```python
from build123d import *

# Parameters (mm, degrees)
ESBO_O2_W                  = 8.2
ESBO_O2_H                  = 30.460387467
RESSALTO_EXTRUS_O1_DEPTH   = 3
RESSALTO_EXTRUS_O1_2_DEPTH = 3
RESSALTO_EXTRUS_O2_REACH   = 32.935
ESBO_O3_W                  = 3
ESBO_O3_H                  = 6.088150409
ESBO_O4_W                  = 12.8
ESBO_O4_H                  = 2.7
RESSALTO_EXTRUS_O3_DEPTH   = 10
ESBO_O5_W                  = 8.2
ESBO_O5_H                  = 4.5
RESSALTO_EXTRUS_O4_DEPTH   = 16
CORTE_EXTRUS_O1_DEPTH      = 34.348189118
CORTE_EXTRUS_O1_DEPTH_BACK = 34.348189118
ESBO_O6_R                  = 1.6
ESBO_O7_R                  = 3
CORTE_EXTRUS_O2_DEPTH      = 2.5
ESBO_O8_R                  = 1.05
CORTE_EXTRUS_O3_DEPTH      = 32.131124741
FILETE1_R                  = 3
ESBO_O9_W                  = 1.2
ESBO_O9_H                  = 3.148787123
CORTE_EXTRUS_O4_DEPTH      = 2.7
FILETE2_R                  = 3
CORTE_EXTRUS_O5_DEPTH      = 1.8
ESBO_O13_W                 = 2.7
ESBO_O13_H                 = 3.148787123
CORTE_EXTRUS_O7_DEPTH      = 1.2


with BuildPart() as part:
    # Esbo_o2 → Ressalto-extrus_o1 (new body)
    with BuildSketch(Plane(origin=(0, 0, -1), x_dir=(-1, 0, 0), z_dir=(0, 0, -1))):
        with Locations((10.5, -7.130193734)):
            Rectangle(ESBO_O2_W, ESBO_O2_H)
    extrude(amount=RESSALTO_EXTRUS_O1_DEPTH)


with BuildPart() as body_2:
    # Esbo_o2 → Ressalto-extrus_o1 2 (new body)
    with BuildSketch(Plane(origin=(0, 0, -1), x_dir=(-1, 0, 0), z_dir=(0, 0, -1))):
        with Locations((-10.5, -7.130193734)):
            Rectangle(ESBO_O2_W, ESBO_O2_H)
    extrude(amount=RESSALTO_EXTRUS_O1_2_DEPTH)

    # Esbo_o3 → Ressalto-extrus_o2 (add, up to next)
    with BuildSketch(Plane(origin=(-6.4, 0, 0), x_dir=(0, 0, -1), z_dir=(1, 0, 0)), mode=Mode.PRIVATE) as ressalto_extrus_o2_sk1:
        with Locations((2.5, -19.316312263)):
            Rectangle(ESBO_O3_W, ESBO_O3_H)
    ressalto_extrus_o2_tool1 = extrude(ressalto_extrus_o2_sk1.sketch, amount=RESSALTO_EXTRUS_O2_REACH, mode=Mode.PRIVATE) - body_2.part

    add(part.part)  # Ressalto-extrus_o2 merges part
    add(ressalto_extrus_o2_tool1.solids().sort_by_distance((-6.4, -19.316312, -2.5))[0])

    # Esbo_o4 → Ressalto-extrus_o3 (add)
    with BuildSketch(Plane.XY.offset(-1)):
        with Locations((0, -21.010387467)):
            Rectangle(ESBO_O4_W, ESBO_O4_H)
    extrude(amount=RESSALTO_EXTRUS_O3_DEPTH)

    # Esbo_o5 → Ressalto-extrus_o4 (add)
    with BuildSketch(Plane.XY.offset(-1)):
        with Locations((-10.5, -20.110387467)):
            Rectangle(ESBO_O5_W, ESBO_O5_H)
        with Locations((10.5, -20.110387467)):
            Rectangle(ESBO_O5_W, ESBO_O5_H)
    extrude(amount=RESSALTO_EXTRUS_O4_DEPTH)

    # Esbo_o6 → Corte-extrus_o1 (cut, two sides: drawn at the far end of the back side and taken through both)
    with BuildSketch(Plane(origin=(0, -17.860387467, 0), x_dir=(1, 0, 0), z_dir=(0, 1, 0)).offset(-CORTE_EXTRUS_O1_DEPTH_BACK)):
        with Locations(Location((0, -4, 0), (0, 0, 270))):
            Circle(ESBO_O6_R)
        with Locations(Location((10.5, -10.5, 0), (0, 0, 270))):
            Circle(ESBO_O6_R)
        with Locations(Location((-10.5, -10.5, 0), (0, 0, 270))):
            Circle(ESBO_O6_R)
    extrude(amount=CORTE_EXTRUS_O1_DEPTH + CORTE_EXTRUS_O1_DEPTH_BACK, mode=Mode.SUBTRACT)

    # Esbo_o7 → Corte-extrus_o2 (cut)
    with BuildSketch(Plane(origin=(0, -17.860387467, 0), x_dir=(1, 0, 0), z_dir=(0, 1, 0))):
        with Locations(Location((10.5, -10.5, 0), (0, 0, 270))):
            Circle(ESBO_O7_R)
        with Locations(Location((-10.5, -10.5, 0), (0, 0, 270))):
            Circle(ESBO_O7_R)
    extrude(amount=-CORTE_EXTRUS_O2_DEPTH, mode=Mode.SUBTRACT)

    # Esbo_o8 → Corte-extrus_o3 (cut, through all)
    with BuildSketch(Plane.XY.offset(-1)):
        with Locations((-10.5, 2.1)):
            Circle(ESBO_O8_R)
        with Locations((10.5, 2.1)):
            Circle(ESBO_O8_R)
        with Locations((10.5, -10.2)):
            Circle(ESBO_O8_R)
        with Locations((-10.5, -10.2)):
            Circle(ESBO_O8_R)
    extrude(amount=-CORTE_EXTRUS_O3_DEPTH, mode=Mode.SUBTRACT)

    # Filete1
    filete1_edges = [body_2.edges().sort_by_distance(p)[0] for p in [
        (6.4, -16.272237058, -2.5),
        (-6.4, -16.272237058, -2.5),
    ]]
    fillet(filete1_edges, radius=FILETE1_R)

    # Esbo_o9 → Corte-extrus_o4 (cut)
    with BuildSketch(Plane.ZY.offset(-6.4)):
        with Locations((-1.6, -8.245598841)):
            Rectangle(ESBO_O9_W, ESBO_O9_H)
    extrude(amount=-CORTE_EXTRUS_O4_DEPTH, mode=Mode.SUBTRACT)

    # Filete2
    filete2_edges = [body_2.edges().sort_by_distance(p)[0] for p in [
        (-10.5, -17.860387467, -1),
        (10.5, -17.860387467, -1),
    ]]
    fillet(filete2_edges, radius=FILETE2_R)

    # Esbo_o10 → Corte-extrus_o5 (cut)
    with BuildSketch(Plane(origin=(0, 0, -4), x_dir=(-1, 0, 0), z_dir=(0, 0, -1))):
        Polygon((12.809401077, 2.1), (11.654700538, 4.1), (9.345299462, 4.1), (8.190598923, 2.1), (9.345299462, 0.1), (11.654700538, 0.1), align=None)
        Polygon((12.809401077, -10.2), (11.654700538, -8.2), (9.345299462, -8.2), (8.190598923, -10.2), (9.345299462, -12.2), (11.654700538, -12.2), align=None)
        Polygon((-11.654700538, -12.2), (-12.809401077, -10.2), (-11.654700538, -8.2), (-9.345299462, -8.2), (-8.190598923, -10.2), (-9.345299462, -12.2), align=None)
        Polygon((-11.654700538, 0.1), (-12.809401077, 2.1), (-11.654700538, 4.1), (-9.345299462, 4.1), (-8.190598923, 2.1), (-9.345299462, 0.1), align=None)
    extrude(amount=-CORTE_EXTRUS_O5_DEPTH, mode=Mode.SUBTRACT)

    # Esbo_o13 → Corte-extrus_o7 (cut)
    with BuildSketch(Plane.XY.offset(-1)):
        with Locations((7.75, -8.245598841)):
            Rectangle(ESBO_O13_W, ESBO_O13_H)
        with Locations((7.75, 8.245598841)):
            Rectangle(ESBO_O13_W, ESBO_O13_H)
        with Locations((-7.75, 8.245598841)):
            Rectangle(ESBO_O13_W, ESBO_O13_H)
        with Locations((-7.75, -8.245598841)):
            Rectangle(ESBO_O13_W, ESBO_O13_H)
    extrude(amount=-CORTE_EXTRUS_O7_DEPTH, mode=Mode.SUBTRACT)


solid = body_2.part
```
The model under review builds one solid part; all positions refer to its coordinate system, in mm. A direction names the side the tool comes from. Give positions to 0.01 mm unless a question says otherwise; leave off trailing zeros. Write each loop counter-clockwise with the first axis right and the second up, starting at its lowest first coordinate (ties: lowest second). Pieces come first, ordered by that corner, then holes.
(1) Tool access review of faces 4 (the flat face through (1.3, -19.66, 2.8)), 5 (the flat face through (12.224, 1.086, -3.113)), 6 (the flat face through (-11, -17.86, 7)), 7 (the cylindrical face through (-9.5, -9.88, -1.59)), 8 (the cylindrical face through (12.53, -19.09, 8.29)): name each direction out of +Z, -Z, +X, -X, +Y, -Y from which nothing blocks a thin tool from reaching the whole face with its end or side.
(2) The part is to be moulded in two halves that separate along X. For faces 1 (the flat face through (-11, -20, 15)), 2 (the flat face through (-9.1, -8, -2)), 3 (the flat face through (-14.6, -13, -2)), say which applies: released by +X, released by -X, zero draft, split by the parting line, or undercut.
(3) Consider section A-A, the plane x = -10.5. Give the number of separate pieces and of enclosed holes in the cut face, and give its area (3 significant figures).
(4) For P1, Ø2.5, axis at x = -10.5, y = -10.2, coming from the +Z side; P2, Ø3, axis at x = 3.5, z = 13, coming from the -Y side; P3, Ø3, axis at x = 1.5, y = -20.5, coming from the +Z side; P4, Ø6.5, axis at x = -12.5, z = 6.5, coming from the +Y side, all flat-tipped, find the tip position at first contact; note any pin that passes through.
(5) To check wall thickness, follow L1, parallel to X at y = -21.7, z = 10.5; L2, parallel to X at y = -19.65, z = 10.5; L3, parallel to Y at x = 10.5, z = -1.6. State the ranges of each line that lie inside material, in increasing order.
(6) Consider section C-C, the plane y = -19. Give the boundary of the cut face in (x, z), and give its area (3 significant figures).
(7) Consider section B-B, the plane z = 4. Give the boundary of the cut face in (x, y), and give its area (3 significant figures).
(8) Consider section D-D, the plane y = -5.5. Give the boundary of the cut face in (x, z), and give its area (3 significant figures).
Returned:
1. face 4: +Z, +Y
1. face 5: -Z
1. face 6: +Z, +X, -X, +Y
1. face 7: +Z, -Z
1. face 8: +Y
2. face 1: zero draft
2. face 2: undercut
2. face 3: released by -X
3. separate pieces: 4
3. enclosed holes: 0
3. area: 124 mm2
4. P1: stops at z = -1
4. P2: passes through
4. P3: stops at z = 9
4. P4: stops at y = -17.86
5. L1: x = -14.6 to -12.1, -8.9 to -6.4, 6.4 to 8.9, 12.1 to 14.6
5. L2: x = -14.6 to -13.5, -7.5 to -6.4, 6.4 to 7.5, 13.5 to 14.6
5. L3: y = -22.36 to -11.25, -9.15 to 1.05, 3.15 to 8.1
6. outline: (-14.6, -4) - (14.6, -4) - (14.6, 15) - (6.4, 15) - (6.4, -1) - (-6.4, -1) - (-6.4, 15) - (-14.6, 15) - close; hole circle Ø6 at (-10.5, 10.5); hole circle Ø6 at (10.5, 10.5)
6. area: 293 mm2
7. outline: (-14.6, -22.36) - (-1.6, -22.36) - (-1.6, -19.66) - (-6.4, -19.66) - (-6.4, -17.86) - (-14.6, -17.86) - close; (1.6, -22.36) - (14.6, -22.36) - (14.6, -17.86) - (6.4, -17.86) - (6.4, -19.66) - (1.6, -19.66) - close
7. area: 99.7 mm2
8. outline: (-14.6, -4) - (-6.4, -4) - (-6.4, -1) - (-14.6, -1) - close; (6.4, -4) - (14.6, -4) - (14.6, -1) - (6.4, -1) - close
8. area: 49.2 mm2
